Autodesk Inventor part; units mm, degrees
ref_plane "YZ Plane" through (0, 0, 0) normal (1, 0, 0) x (0, 1, 0)
ref_plane "XZ Plane" through (0, 0, 0) normal (0, 1, 0) x (-1, 0, 0)
ref_plane "XY Plane" through (0, 0, 0) normal (0, 0, 1) x (1, 0, 0)
sketch "Sketch1" plane through (0, 0, 0) normal (0, 1, 0) x (-1, 0, 0)
  line L0 (10.5, 0) -> (-10.5, 0)
  line L1 (0, -42) -> (0, 42)
  line L2 (7.5, -30) -> (-7.5, -30)
  line L3 (-7.5, -30) -> (-7.5, 30)
  line L4 (-7.5, 30) -> (7.5, 30)
  line L5 (7.5, 30) -> (7.5, -30)
  point P0 (0, 0)
  dimension "d0" = 15
  dimension "d1" = 60
extrude "Extrusion1" add sketch "Sketch1" along normal blind 2
fillet "Fillet1" radius 6 4 edges at (7.5, 1, -30) (-7.5, 1, -30) (-7.5, 1, 30) (7.5, 1, 30)
sketch "Sketch5" plane through (0, 2, 0) normal (0, 1, 0) x (1, 0, 0)
  arc A0 (1.5, -30) -> (7.5, -24) centre (1.5, -24) ccw
  line L0 (7.5, -24) -> (7.5, 24)
  arc A1 (7.5, 24) -> (1.5, 30) centre (1.5, 24) ccw
  line L1 (1.5, 30) -> (-1.5, 30)
  arc A2 (-1.5, 30) -> (-7.5, 24) centre (-1.5, 24) ccw
  line L2 (-7.5, 24) -> (-7.5, -24)
  arc A3 (-7.5, -24) -> (-1.5, -30) centre (-1.5, -24) ccw
  line L3 (-1.5, -30) -> (1.5, -30)
  point P0 (0, 0)
  point P1 (0, 0)
hole "Hole3" at (0, 2, 0) direction (0, -1, 0) diameter 4 end through all
sketch "Sketch6" plane through (0, 2, 0) normal (0, 1, 0) x (1, 0, 0)
  circle A0 centre (0, 0) radius 2
  arc A1 (1.5, -30) -> (7.5, -24) centre (1.5, -24) ccw
  line L0 (7.5, -24) -> (7.5, 24)
  arc A2 (7.5, 24) -> (1.5, 30) centre (1.5, 24) ccw
  line L1 (1.5, 30) -> (-1.5, 30)
  arc A3 (-1.5, 30) -> (-7.5, 24) centre (-1.5, 24) ccw
  line L2 (-7.5, 24) -> (-7.5, -24)
  arc A4 (-7.5, -24) -> (-1.5, -30) centre (-1.5, -24) ccw
  line L3 (-1.5, -30) -> (1.5, -30)
  line L4 (0, 43.7397) -> (0, -43.7397)
  line L5 (-12.2397, 0) -> (12.2397, 0)
  point P0 (0, 22)
  point P1 (0, -22)
  dimension "d41" = 8
  dimension "d42" = 8
hole "Hole4" at (0, 2, -22) at (0, 2, 22) direction (0, -1, 0) diameter 7 end through all
properties part number "femur_v5"
Verification items for the finished model (mm, model axes). Give positions to 0.01 mm unless a question says otherwise; leave off trailing zeros. Order: outer loops, then holes, each group sorted by start corner. A loop starts at its lowest first (then second) coordinate and runs counter-clockwise, first axis right, second up. Notation, with made-up numbers: M 71.5,6.25 L 111.5,6.25 A19 cw 111.5,33.25 Z; hole C 19,76 d7. An arc over 180 degrees is marked long. Use one line per item in the form item = value. Start each with the question number.
Q1. Go/stop test with flat-tipped pins: pin 1 Ø5.5 at (x, z) = (0, -22) entering from +Y; pin 2 Ø1 at (x, y) = (-2.5, 1) entering from +Z. Record where each tip stops, or that it passes through.
Q2. Mould release check, pull along X, two halves, no side actions. Record for faces 1 (the flat face through (0, 1, 30)), 2 (the cylindrical face through (5.696, 1.014, 28.289)), 3 (the cylindrical face through (-1.05, 0.99, -18.66)): +X half, -X half, draft (parallel to the pull), parting line (faces both ways), or undercut.
Q3. Section check B-B (x = 0). Enter the section's corners in (y, z).
Q4. Section check D-D (z = 22). Enter the section's corners in (x, y).
Q5. Section check A-A (z = 0). Enter the section's corners in (x, y).
Q6. Scan lines: line 1 along Z through (x, y) = (0, 1.55); line 2 along X through (y, z) = (0.7, -22); line 3 along Z through (x, y) = (-0.75, 1.5). Record each from-to range of solid material in increasing order. Write a range as [from, to].
Q7. Section check C-C (y = 1). Enter the section's corners in (x, z).
Evaluation:
q1.pin_1 = through
q1.pin_2 = 29.98
q2.face_1 = draft
q2.face_2 = +X half
q2.face_3 = undercut
q3.outline = M 0,-30 L 2,-30 L 2,-25.5 L 0,-25.5 Z; M 0,-18.5 L 2,-18.5 L 2,-2 L 0,-2 Z; M 0,2 L 2,2 L 2,18.5 L 0,18.5 Z; M 0,25.5 L 2,25.5 L 2,30 L 0,30 Z
q4.outline = M -7.5,0 L -3.5,0 L -3.5,2 L -7.5,2 Z; M 3.5,0 L 7.5,0 L 7.5,2 L 3.5,2 Z
q5.outline = M -7.5,0 L -2,0 L -2,2 L -7.5,2 Z; M 2,0 L 7.5,0 L 7.5,2 L 2,2 Z
q6.line_1 = [-30, -25.5], [-18.5, -2], [2, 18.5], [25.5, 30]
q6.line_2 = [-7.5, -3.5], [3.5, 7.5]
q6.line_3 = [-30, -25.42], [-18.58, -1.85], [1.85, 18.58], [25.42, 30]
q7.outline = M -7.5,-24 A6 ccw -1.5,-30 L 1.5,-30 A6 ccw 7.5,-24 L 7.5,24 A6 ccw 1.5,30 L -1.5,30 A6 ccw -7.5,24 Z; hole C 0,-22 d7; hole C 0,22 d7; hole C 0,0 d4
